```python
from build123d import *

# Parameters (mm, degrees)
SKETCH1_W                                           = 117.86
SKETCH1_H                                           = 73.41
SKETCH1_R                                           = 1.6
BOSS_EXTRUDE1_DEPTH                                 = 4
SKETCH1_3_W                                         = 16
SKETCH1_3_H                                         = 6
BOSS_EXTRUDE2_DEPTH                                 = 30
CUT_EXTRUDE1_REACH                                  = 107.41
SKETCH2_R                                           = 3.2639
CSK_FOR_1_4_FLAT_HEAD_SOCKET_CAP_SCREW1_D           = 6.5278
CSK_FOR_1_4_FLAT_HEAD_SOCKET_CAP_SCREW1_CSINK_D     = 13.4874
CSK_FOR_1_4_FLAT_HEAD_SOCKET_CAP_SCREW1_CSINK_ANGLE = 82
FILLET1_R                                           = 1
CSK_FOR_M3_SFHCS1_D                                 = 3.2
CSK_FOR_M3_SFHCS1_CSINK_D                           = 6.92
CSK_FOR_M3_SFHCS1_CSINK_ANGLE                       = 90
CHAMFER1_SIZE                                       = 0.3


with BuildPart() as part:
    # Sketch1 → Boss-Extrude1 (new body)
    with BuildSketch(Plane.XY):
        Polygon((-68.93, 45.21), (-68.93, -60.2), (-52.93, -60.2), (-52.93, -48.2), (-8, -48.2), (-8, -60.2), (8, -60.2), (8, -48.2), (52.93, -48.2), (52.93, -60.2), (68.93, -60.2), (68.93, 45.21), align=None)
        with Locations((0, -1.495)):
            Rectangle(SKETCH1_W, SKETCH1_H, mode=Mode.SUBTRACT)
        with Locations((-63.93, 40.21)):
            Circle(SKETCH1_R, mode=Mode.SUBTRACT)
        with Locations((-63.93, -43.2)):
            Circle(SKETCH1_R, mode=Mode.SUBTRACT)
        with Locations((63.93, 40.21)):
            Circle(SKETCH1_R, mode=Mode.SUBTRACT)
        with Locations((63.93, -43.2)):
            Circle(SKETCH1_R, mode=Mode.SUBTRACT)
    extrude(amount=BOSS_EXTRUDE1_DEPTH)

    # Sketch1_3 → Boss-Extrude2 (add)
    with BuildSketch(Plane.XY):
        with Locations((-60.93, -57.2)):
            Rectangle(SKETCH1_3_W, SKETCH1_3_H)
        with Locations((0, -57.2)):
            Rectangle(SKETCH1_3_W, SKETCH1_3_H)
        with Locations((60.93, -57.2)):
            Rectangle(SKETCH1_3_W, SKETCH1_3_H)
    extrude(amount=-BOSS_EXTRUDE2_DEPTH)

    # Sketch2 → Cut-Extrude1 (cut, up to next)
    with BuildSketch(Plane.XZ.offset(60.2), mode=Mode.PRIVATE) as cut_extrude1_sk1:
        with Locations((-60.93, -22)):
            Circle(SKETCH2_R)
    cut_extrude1_tool1 = extrude(cut_extrude1_sk1.sketch, amount=-CUT_EXTRUDE1_REACH, mode=Mode.PRIVATE) & part.part
    add(cut_extrude1_tool1.solids().sort_by_distance((-60.93, -60.2, -22))[0], mode=Mode.SUBTRACT)
    # Sketch2 → Cut-Extrude1 (cut, up to next)
    with BuildSketch(Plane.XZ.offset(60.2), mode=Mode.PRIVATE) as cut_extrude1_sk2:
        with Locations((0, -22)):
            Circle(SKETCH2_R)
    cut_extrude1_tool2 = extrude(cut_extrude1_sk2.sketch, amount=-CUT_EXTRUDE1_REACH, mode=Mode.PRIVATE) & part.part
    add(cut_extrude1_tool2.solids().sort_by_distance((0, -60.2, -22))[0], mode=Mode.SUBTRACT)
    # Sketch2 → Cut-Extrude1 (cut, up to next)
    with BuildSketch(Plane.XZ.offset(60.2), mode=Mode.PRIVATE) as cut_extrude1_sk3:
        with Locations((60.93, -22)):
            Circle(SKETCH2_R)
    cut_extrude1_tool3 = extrude(cut_extrude1_sk3.sketch, amount=-CUT_EXTRUDE1_REACH, mode=Mode.PRIVATE) & part.part
    add(cut_extrude1_tool3.solids().sort_by_distance((60.93, -60.2, -22))[0], mode=Mode.SUBTRACT)

    # CSK for 1_4 Flat Head Socket Cap Screw1 (through all)
    with Locations(Plane(origin=(0, -60.2, 0), x_dir=(-1, 0, 0), z_dir=(0, -1, 0))):
        with Locations((60.93, 22), (0, 22), (-60.93, 22)):
            CounterSinkHole(CSK_FOR_1_4_FLAT_HEAD_SOCKET_CAP_SCREW1_D / 2, CSK_FOR_1_4_FLAT_HEAD_SOCKET_CAP_SCREW1_CSINK_D / 2, counter_sink_angle=CSK_FOR_1_4_FLAT_HEAD_SOCKET_CAP_SCREW1_CSINK_ANGLE)

    # Fillet1
    fillet1_edges = [part.edges().sort_by_distance(p)[0] for p in [
        (52.93, -60.2, -13),
        (8, -60.2, -13),
        (-8, -60.2, -13),
        (-52.93, -60.2, -13),
        (-68.93, -60.2, -13),
        (-68.93, 45.21, 2),
        (68.93, 45.21, 2),
        (68.93, -60.2, -13),
        (-52.93, -54.2, -15),
        (-60.93, -60.2, -30),
        (-68.93, -57.2, -30),
        (-68.93, -54.2, -15),
        (-52.93, -57.2, -30),
        (-60.93, -54.2, -30),
        (-8, -54.2, -15),
        (8, -54.2, -15),
        (0, -60.2, -30),
        (-8, -57.2, -30),
        (0, -54.2, -30),
        (8, -57.2, -30),
        (52.93, -54.2, -15),
        (68.93, -54.2, -15),
        (52.93, -57.2, -30),
        (60.93, -54.2, -30),
        (68.93, -57.2, -30),
        (60.93, -60.2, -30),
    ]]
    fillet(fillet1_edges, radius=FILLET1_R)

    # CSK for M3 SFHCS1 (through all)
    with Locations(Plane(origin=(0, 0, 0), x_dir=(-1, 0, 0), z_dir=(0, 0, -1))):
        with Locations((63.93, 40.21), (63.93, -43.2), (-63.93, -43.2), (-63.93, 40.21)):
            CounterSinkHole(CSK_FOR_M3_SFHCS1_D / 2, CSK_FOR_M3_SFHCS1_CSINK_D / 2, counter_sink_angle=CSK_FOR_M3_SFHCS1_CSINK_ANGLE)

    # Chamfer1
    chamfer1_edges = [part.edges().sort_by_distance(p)[0] for p in [
        (0, 35.21, 4),
        (-68.93, -7.495, 4),
        (-60.93, -60.2, 4),
        (0, -60.2, 4),
        (60.93, -60.2, 4),
        (68.93, -7.495, 4),
        (0, 45.21, 4),
        (68.637106781, 44.917106781, 4),
        (-68.637106781, 44.917106781, 4),
        (-53.222893219, -59.907106781, 4),
        (-68.637106781, -59.907106781, 4),
        (-7.707106781, -59.907106781, 4),
        (7.707106781, -59.907106781, 4),
        (53.222893219, -59.907106781, 4),
        (68.637106781, -59.907106781, 4),
        (-52.93, -53.7, 4),
        (-30.465, -48.2, 4),
        (-8, -53.7, 4),
        (8, -53.7, 4),
        (30.465, -48.2, 4),
        (52.93, -53.7, 4),
        (58.93, -1.495, 4),
        (0, -38.2, 4),
        (-58.93, -1.495, 4),
    ]]
    chamfer(chamfer1_edges, length=CHAMFER1_SIZE)


solid = part.part
```
For this review, take the finished solid that the model builds, in its own axes (mm). A direction names the side the tool comes from. Coordinates: 2 decimals unless noted, no trailing zeros. Write each loop counter-clockwise with the first axis right and the second up, starting at its lowest first coordinate (ties: lowest second). Pieces come first, ordered by that corner, then holes. Notation, with made-up numbers: (82, 41.25) -> (90, 41.25) arc R36 cw to (90, 77.25) -> close; hole circle Ø8 at (-32.75, 10.25). An arc over 180 degrees is marked (long way). Put each result on its own line as item: value.
Q1. Take a section at C-C, the plane z = -3.5. State the section outline as (x, y) points.
From the geometry:
outline: (-68.93, -59.2) arc R1 ccw to (-67.93, -60.2) -> (-53.93, -60.2) arc R1 ccw to (-52.93, -59.2) -> (-52.93, -55.2) arc R1 ccw to (-53.93, -54.2) -> (-67.93, -54.2) arc R1 ccw to (-68.93, -55.2) -> close; (-8, -59.2) arc R1 ccw to (-7, -60.2) -> (7, -60.2) arc R1 ccw to (8, -59.2) -> (8, -55.2) arc R1 ccw to (7, -54.2) -> (-7, -54.2) arc R1 ccw to (-8, -55.2) -> close; (52.93, -59.2) arc R1 ccw to (53.93, -60.2) -> (67.93, -60.2) arc R1 ccw to (68.93, -59.2) -> (68.93, -55.2) arc R1 ccw to (67.93, -54.2) -> (53.93, -54.2) arc R1 ccw to (52.93, -55.2) -> close
Q2. Take a section at A-A, the plane y = 1. State the section outline as (x, z) points, then the cut area to 3 significant figures.
From the geometry:
outline: (-68.93, 0) -> (-58.93, 0) -> (-58.93, 3.7) -> (-59.23, 4) -> (-68.63, 4) -> (-68.93, 3.7) -> close; (58.93, 0) -> (68.93, 0) -> (68.93, 3.7) -> (68.63, 4) -> (59.23, 4) -> (58.93, 3.7) -> close
area: 79.8 mm2
Q3. Tool access review of faces 1 (the flat face through (1, 45.21, 2)), 2 (the flat face through (-31, -48.2, 2)), 3 (the flat face through (-1, 35.21, 2)): name each direction out of +Z, -Z, +X, -X, +Y, -Y from which nothing blocks a thin tool from reaching the whole face with its end or side.
From the geometry:
face 1: +Z, -Z, +X, -X, +Y
face 2: +Z, -Z, -Y
face 3: +Z, -Z
Q4. Clearance check with flat-ended pins moving along their axes: pin 1 Ø4 at (x, z) = (-33.5, 1.5) entering from -Y; pin 2 Ø3.5 at (y, z) = (-53, -17.5) entering from -X; pin 3 Ø11 at (x, z) = (64, -10.5) entering from +Y. State where each tip first meets the part, or that it passes through.
From the geometry:
pin 1: stops at y = -48.2
pin 2: stops at x = -68.82
pin 3: stops at y = -54.2
Q5. Take a section at D-D, the plane x = 0. State the section outline as (y, z) points, then the cut area to 3 significant figures.
From the geometry:
outline: (-60.2, -29) arc R1 ccw to (-59.2, -30) -> (-55.2, -30) arc R1 ccw to (-54.2, -29) -> (-54.2, -25.26) -> (-56.2, -25.26) -> (-60.2, -28.74) -> close; (-60.2, -15.26) -> (-56.2, -18.74) -> (-54.2, -18.74) -> (-54.2, 0) -> (-38.2, 0) -> (-38.2, 3.7) -> (-38.5, 4) -> (-59.9, 4) -> (-60.2, 3.7) -> close; (35.21, 0) -> (45.21, 0) -> (45.21, 3.7) -> (44.91, 4) -> (35.51, 4) -> (35.21, 3.7) -> close
area: 254 mm2
Q6. Take a section at B-B, the plane x = 38.5. State the section outline as (y, z) points, then the cut area to 3 significant figures.
From the geometry:
outline: (-48.2, 0) -> (-38.2, 0) -> (-38.2, 3.7) -> (-38.5, 4) -> (-47.9, 4) -> (-48.2, 3.7) -> close; (35.21, 0) -> (45.21, 0) -> (45.21, 3.7) -> (44.91, 4) -> (35.51, 4) -> (35.21, 3.7) -> close
area: 79.8 mm2
Q7. Wall thickness on L1, parallel to X at y = -43.2, z = 3.55; L2, parallel to Z at x = 60.93, y = -55.7; L3, parallel to Y at x = 24, z = 2.5: over which ranges is each line inside the solid? List them lowest first.
From the geometry:
L1: x = -68.93 to -65.53, -62.33 to 62.33, 65.53 to 68.93
L2: z = -30 to -25.26, -18.74 to 4
L3: y = -48.2 to -38.2, 35.21 to 45.21
Q8. The part is to be moulded in two halves that separate along Y. For faces 4 (the conical face through (-0.74, -56.39, -18.65)), 5 (the cylindrical face through (65.41, 39.6, 2.92)), 6 (the flat face through (-1, -42, 4)), say which applies: +Y half, -Y half, draft (parallel to the pull), parting line (faces both ways), or undercut.
From the geometry:
face 4: -Y half
face 5: undercut
face 6: draft
